Here's how the part is built. I have some questions about the finished solid (model axes, mm). A direction names the side the tool comes from. Coordinates: 2 decimals unless noted, no trailing zeros. Order: outer loops, then holes, each group sorted by start corner. A loop starts at its lowest first (then second) coordinate and runs counter-clockwise, first axis right, second up.
```python
from build123d import *

# Parameters (mm, degrees)
EXTRUDE018_DEPTH = 60
EXTRUDE037_DEPTH = 26.5


with BuildPart() as body014:
    # Sketch022 → Extrude018 (new body)
    with BuildSketch(Plane.XZ.offset(46)):
        Polygon((-21, 7.5), (-102, 7.5), (-102, -12), (-94, -20), (-26, -20), (-21, -15), align=None)
    extrude(amount=-EXTRUDE018_DEPTH)


with BuildPart() as cut007:
    # Sketch044 → Extrude037 (new body)
    with BuildSketch(Plane.XY.offset(-25.5)):
        Polygon((-11, -1), (-23.012985, -1), (-100.025965, 1.000337), (-100, 2), (-23, 0), (-11, 0), align=None)
    extrude(amount=EXTRUDE037_DEPTH)

    # Cut007: cut Body014
    add(body014.part, mode=Mode.SUBTRACT)


solid = cut007.part
```
Q1. For faces 1 (the flat face through (-60.5, 0.4, -20)), 2 (the flat face through (-55, 0, -25.5)), 3 (the flat face through (-16, 0, -12)), which set-ups out of +Z, -Z, +X, -X, +Y, -Y let a thin tool reach every point of the face, with its end or its side?
Q2. Will these pins go through, and if not, where does the flat tip stop? pin 1 (1.1 mm diameter, centred on y = -0.5, z = -6, fed in from -X); pin 2 (1.5 mm diameter, centred on y = -0.5, z = -17, fed in from -X); pin 3 (6 mm diameter, centred on x = -20, z = -9.5, fed in from +Y).
Q3. If we section it at D-D on z = -1.75: Write out the boundary of the cut face in (x, y), then the cut area to 3 significant figures.
Q4. I need wall thicknesses on L1, parallel to Z at x = -61, y = 0.7; L2, parallel to Y at x = -16, z = -18.5; L3, parallel to X at y = -0.4, z = -13.75. Which ranges of each line are inside material? Lowest first, please.
Q5. If we section it at A-A on z = -19.25: Write out the boundary of the cut face in (x, y).
Q6. If we section it at C-C on z = -23.25: Write out the boundary of the cut face in (x, y).
Q7. If we section it at B-B on x = -16.5: Write out the boundary of the cut face in (y, z), then the cut area to 3 significant figures.
Reply:
1. face 1: +Z, +Y, -Y
1. face 2: -Z, +X, -X, +Y, -Y
1. face 3: +Z, -Z, +X, +Y
2. pin 1: stops at x = -21
2. pin 2: stops at x = -23.75
2. pin 3: stops at y = 0
3. outline: (-21, -1) - (-11, -1) - (-11, 0) - (-21, 0) - close
3. area: 10.0 mm2
4. L1: z = -25.5 to -20
4. L2: y = -1 to 0
4. L3: x = -21 to -11
5. outline: (-100.03, 1) - (-94.75, 0.86) - (-94.75, 1.86) - (-100, 2) - close; (-25.25, -0.94) - (-23.01, -1) - (-11, -1) - (-11, 0) - (-23, 0) - (-25.25, 0.06) - close
6. outline: (-100.03, 1) - (-23.01, -1) - (-11, -1) - (-11, 0) - (-23, 0) - (-100, 2) - close
7. outline: (-1, -25.5) - (0, -25.5) - (0, 1) - (-1, 1) - close
7. area: 26.5 mm2
